```python
from build123d import *

# Parameters (mm, degrees)
EXTRUDE_START          = 25
EXTRUDE_1_DEPTH        = 50
SKETCH_4_R             = 4.5
CUT_EXTRUDE_1_DEPTH    = 85.274847968
SKETCH_6_R             = 3
CUT_EXTRUDE_2_DEPTH    = 47.238512087
SKETCH_7_R             = 14
CUT_EXTRUDE_3_DEPTH    = 47.238512087
SKETCH_9_W             = 50
SKETCH_9_H             = 9.8
CUT_EXTRUDE_4_DEPTH    = 47.238512087
CUT_EXTRUDE_1983_DEPTH = 42.051674753
FILLET_1_R             = 2.5


with BuildPart() as part:
    # 草图3 → 凸台-拉伸1 (new body)
    with BuildSketch(Plane(origin=(0, 0, 0), x_dir=(0, 0, -1), z_dir=(1, 0, 0)).offset(EXTRUDE_START)):
        with BuildLine():
            Line((-76.5, 0), (-76.5, 3))
            Line((-76.5, 3), (-51.55, 3))
            ThreePointArc((-51.55, 3), (-50.100431099, 3.600431099), (-49.5, 5.05))
            Line((-49.5, 5.05), (-49.5, 28))
            Line((-49.5, 28), (-46.5, 28))
            Line((-46.5, 28), (-46.5, 5.05))
            ThreePointArc((-46.5, 5.05), (-47.979110755, 1.479110755), (-51.55, 0))
            Line((-51.55, 0), (-76.5, 0))
        make_face()
    extrude(amount=-EXTRUDE_1_DEPTH)

    # 草图4 → 切除-拉伸1 (cut, through all)
    with BuildSketch(Plane(origin=(0, 3, 0), x_dir=(1, 0, 0), z_dir=(0, 1, 0))):
        with Locations(Location((-16.5, -67, 0), (0, 0, 270))):
            Circle(SKETCH_4_R)
    cut_extrude_1 = extrude(amount=-CUT_EXTRUDE_1_DEPTH, mode=Mode.SUBTRACT)

    # 镜向1: 切除-拉伸1 across plane
    add(cut_extrude_1.mirror(Plane(origin=(0, 0, 0), x_dir=(0, 0, 1), z_dir=(1, 0, 0))), mode=Mode.SUBTRACT)

    # 草图6 → 切除-拉伸2 (cut, through all)
    with BuildSketch(Plane.XY.offset(49.5)):
        with Locations((-16.5, 11.5)):
            Circle(SKETCH_6_R)
    cut_extrude_2 = extrude(amount=-CUT_EXTRUDE_2_DEPTH, mode=Mode.SUBTRACT)

    # 镜向2: 切除-拉伸2 across plane
    add(cut_extrude_2.mirror(Plane(origin=(0, 0, 0), x_dir=(0, 0, 1), z_dir=(1, 0, 0))), mode=Mode.SUBTRACT)

    # 草图7 → 切除-拉伸3 (cut, through all)
    with BuildSketch(Plane.XY.offset(49.5)):
        with Locations((0, 28)):
            Circle(SKETCH_7_R)
    extrude(amount=-CUT_EXTRUDE_3_DEPTH, mode=Mode.SUBTRACT)

    # 草图9 → 切除-拉伸4 (cut, through all)
    with BuildSketch(Plane.XY.offset(49.5)):
        with Locations((0, 23.1)):
            Rectangle(SKETCH_9_W, SKETCH_9_H)
    extrude(amount=-CUT_EXTRUDE_4_DEPTH, mode=Mode.SUBTRACT)

    # 草图8 → Cut-Extrude 1983 (cut, through all)
    with BuildSketch(Plane.XY.offset(49.5)):
        Polygon((-22.5, 18.2), (22.5, 18.2), (25, 6.17), (25, 28), (-25, 28), (-25, 6.17), align=None)
    extrude(amount=-CUT_EXTRUDE_1983_DEPTH, mode=Mode.SUBTRACT)

    # 圆角1
    fillet_1_edges = [part.edges().sort_by_distance(p)[0] for p in [
        (22.5, 18.2, 48),
        (-22.5, 18.2, 48),
    ]]
    fillet(fillet_1_edges, radius=FILLET_1_R)


solid = part.part
```
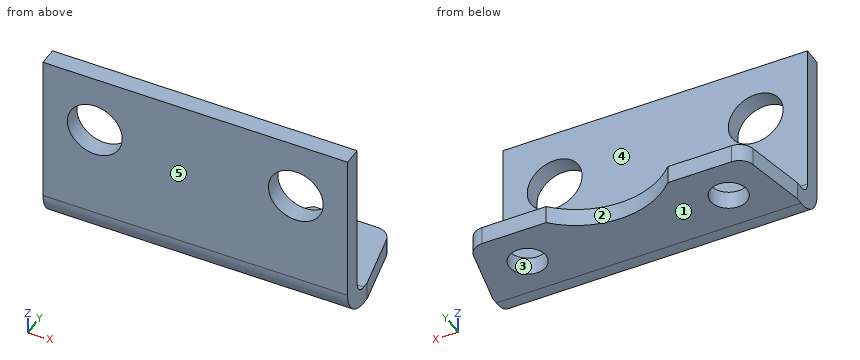
Work out the finished part from the listing and answer in its coordinate system (mm). Face numbers are marked on the shaded views. A direction names the side the tool comes from. Give positions to 0.01 mm unless a question says otherwise; leave off trailing zeros. Write each loop counter-clockwise with the first axis right and the second up, starting at its lowest first coordinate (ties: lowest second). Pieces come first, ordered by that corner, then holes.
(1) Straight lines are drawn through the part: line 1 (X direction, y = 0.7, z = 67); line 2 (Y direction, x = 19, z = 54.75); line 3 (Z direction, x = 22.5, y = 13.25). For each, find the intervals that lie inside material, in ascending order.
Final values:
line 1: x = -25 to -21, -12 to 12, 21 to 25
line 2: y = 0 to 3
line 3: z = 46.5 to 49.5
(2) The part is cut by section A-A on x = 16.5. Write down the section's boundary in (y, z).
Final values:
outline: (0, 51.55) arc R5.05 ccw to (5.05, 46.5) - (8.5, 46.5) - (8.5, 49.5) - (5.05, 49.5) arc R2.05 cw to (3, 51.55) - (3, 62.5) - (0, 62.5) - close; (0, 71.5) - (3, 71.5) - (3, 76.5) - (0, 76.5) - close; (14.5, 46.5) - (18.2, 46.5) - (18.2, 49.5) - (14.5, 49.5) - close
(3) The part is cut by section C-C on y = 15.5. Write down the section's boundary in (x, z), plus the area to 3 significant figures.
Final values:
outline: (-23.06, 46.5) - (-6.3, 46.5) - (-6.3, 49.5) - (-23.06, 49.5) - close; (6.3, 46.5) - (23.06, 46.5) - (23.06, 49.5) - (6.3, 49.5) - close
area: 101 mm2
(4) Which of the six approach directions +Z, -Z, +X, -X, +Y, -Y give full straight-line access (tool end or side, diameter ignored) to the marked faces 4 and 5?
Final values:
face 4: +Z, +X, -X, +Y
face 5: +Z, -Z, +X, -X, -Y
(5) The part is cut by section D-D on x = -11.5. Write down the section's boundary in (y, z), plus the area to 3 significant figures.
Final values:
outline: (0, 51.55) arc R5.05 ccw to (5.05, 46.5) - (18.2, 46.5) - (18.2, 49.5) - (5.05, 49.5) arc R2.05 cw to (3, 51.55) - (3, 76.5) - (0, 76.5) - close
area: 131 mm2
(6) The mould has two halves that part along Y. Classify the marked faces 1, 2 and 3: pulls with the +Y half, pulls with the -Y half, needs draft (parallel to the pull), parting line crosses it, or undercut.
Final values:
face 1: needs draft
face 2: pulls with the +Y half
face 3: undercut
(7) Flat-ended cylindrical pins translate along their axes: pin 1 Ø10 at (y, z) = (4, 59.5) entering from -X; pin 2 Ø5.5 at (x, y) = (-16.5, 11.5) entering from +Z; pin 3 Ø10 at (x, y) = (-5, 14) entering from +Z; pin 4 Ø12.5 at (x, z) = (12.5, 69) entering from +Y. Find the tip coordinate at first contact, or state that the pin passes through.
Final values:
pin 1: stops at x = -25
pin 2: passes through
pin 3: stops at z = 49.5
pin 4: stops at y = 3
(8) The part is cut by section B-B on y = 9.75. Write down the section's boundary in (x, z), plus the area to 3 significant figures.
Final values:
outline: (-24.26, 46.5) - (-18.94, 46.5) - (-18.94, 49.5) - (-24.26, 49.5) - close; (-14.06, 46.5) - (14.06, 46.5) - (14.06, 49.5) - (-14.06, 49.5) - close; (18.94, 46.5) - (24.26, 46.5) - (24.26, 49.5) - (18.94, 49.5) - close
area: 116 mm2
